Here's how the part is built. I have some questions about the finished solid (model axes, mm). Face numbers are marked on the shaded views. A direction names the side the tool comes from. Give positions to 0.01 mm unless a question says otherwise; leave off trailing zeros. Loops run counter-clockwise (first coordinate to the right, second up) from the corner with the lowest first, then second, coordinate; pieces in that order, holes last. Notation, with made-up numbers: (-13.5, 6.5) - (4.5, 6.5) arc R19 ccw to (4.5, 37.5) - close; hole circle Ø2 at (-7, -7). An arc over 180 degrees is marked (long way). Use a Markdown table: item, result.
from build123d import *

# Parameters (mm, degrees)
SKETCH1_R           = 25
SKETCH1_R_2         = 3
BOSS_EXTRUDE1_DEPTH = 12.5
CUT_EXTRUDE2_DEPTH  = 10
CUT_EXTRUDE3_START  = -4.5
SKETCH2_4_R         = 35
SKETCH2_4_R_2       = 25
CUT_EXTRUDE3_DEPTH  = 17


with BuildPart() as part:
    # Sketch1 → Boss-Extrude1 (new, symmetric)
    with BuildSketch(Plane.XY):
        with BuildLine():
            Line((-33, -40), (33, -40))
            ThreePointArc((33, -40), (37.949747468, -37.949747468), (40, -33))
            Line((40, -33), (40, 33))
            ThreePointArc((40, 33), (37.949747468, 37.949747468), (33, 40))
            Line((33, 40), (-33, 40))
            ThreePointArc((-33, 40), (-37.949747468, 37.949747468), (-40, 33))
            Line((-40, 33), (-40, -33))
            ThreePointArc((-40, -33), (-37.949747468, -37.949747468), (-33, -40))
        make_face()
        Circle(SKETCH1_R, mode=Mode.SUBTRACT)
        with Locations((-33, 33)):
            Circle(SKETCH1_R_2, mode=Mode.SUBTRACT)
        with Locations((33, 33)):
            Circle(SKETCH1_R_2, mode=Mode.SUBTRACT)
        with Locations((-33, -33)):
            Circle(SKETCH1_R_2, mode=Mode.SUBTRACT)
        with Locations((33, -33)):
            Circle(SKETCH1_R_2, mode=Mode.SUBTRACT)
    extrude(amount=BOSS_EXTRUDE1_DEPTH, both=True)

    # Sketch2 → Cut-Extrude2 (cut, symmetric)
    with BuildSketch(Plane.XY):
        with BuildLine():
            Line((-40, 33), (-40, 14.361406616))
            ThreePointArc((-40, 14.361406616), (-30.0520382, 30.0520382), (-14.361406616, 40))
            Line((-14.361406616, 40), (-33, 40))
            ThreePointArc((-33, 40), (-37.949747468, 37.949747468), (-40, 33))
        make_face()
        with BuildLine():
            Line((33, 40), (14.361406616, 40))
            ThreePointArc((14.361406616, 40), (30.0520382, 30.0520382), (40, 14.361406616))
            Line((40, 14.361406616), (40, 33))
            ThreePointArc((40, 33), (37.949747468, 37.949747468), (33, 40))
        make_face()
        with BuildLine():
            ThreePointArc((40, -14.361406616), (30.0520382, -30.0520382), (14.361406616, -40))
            Line((14.361406616, -40), (33, -40))
            ThreePointArc((33, -40), (37.949747468, -37.949747468), (40, -33))
            Line((40, -33), (40, -14.361406616))
        make_face()
        with BuildLine():
            ThreePointArc((-14.361406616, -40), (-30.0520382, -30.0520382), (-40, -14.361406616))
            Line((-40, -14.361406616), (-40, -33))
            ThreePointArc((-40, -33), (-37.949747468, -37.949747468), (-33, -40))
            Line((-33, -40), (-14.361406616, -40))
        make_face()
    extrude(amount=CUT_EXTRUDE2_DEPTH, both=True, mode=Mode.SUBTRACT)

    # Sketch2<4> → Cut-Extrude3 (cut)
    with BuildSketch(Plane.XY.offset(CUT_EXTRUDE3_START)):
        Circle(SKETCH2_4_R)
        Circle(SKETCH2_4_R_2, mode=Mode.SUBTRACT)
    extrude(amount=CUT_EXTRUDE3_DEPTH, mode=Mode.SUBTRACT)


solid = part.part
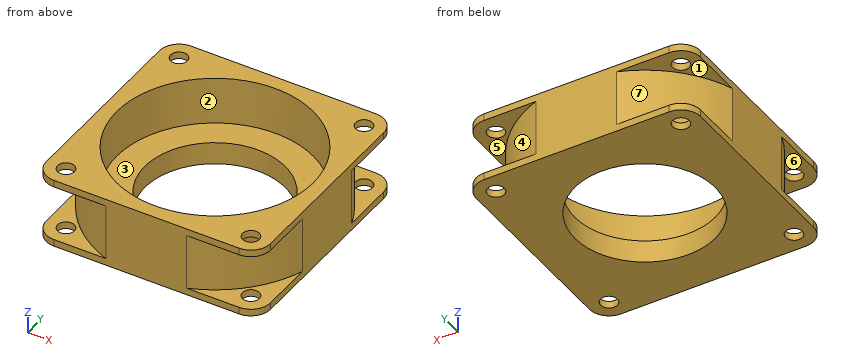
(1) Will these pins go through, and if not, where does the flat tip stop? pin 1 (8 mm diameter, centred on x = 33, y = 33, fed in from -Z); pin 2 (2 mm diameter, centred on y = -24, z = 0.5, fed in from +X); pin 3 (1 mm diameter, centred on y = -27, z = -6.5, fed in from -X); pin 4 (1 mm diameter, centred on y = 15.5, z = -3, fed in from -X).
A:
| item | result |
|---|---|
| pin 1 | z = -12.5 |
| pin 2 | x = 35.74 |
| pin 3 | x = -33.23 |
| pin 4 | x = -39.76 |
(2) On a 3-axis mill with a long thin cutter (end or side, diameter ignored), from which of +Z, -Z, +X, -X, +Y, -Y can I reach the whole of each face in a straight line? I mean the marked faces 5, 6 and 7. Say none if no direction works.
A:
| item | result |
|---|---|
| face 5 | +X, +Y |
| face 6 | -X, -Y |
| face 7 | -X, +Y |
(3) Suppose I cut it at D-D on y = -32. Count the separate pieces of the cut face and the enclosed holes in it, plus the area to 3 significant figures.
A:
| item | result |
|---|---|
| separate pieces | 5 |
| enclosed holes | 0 |
| area | 980 mm2 |
(4) If I drill on line 1 (Y direction, x = 33, z = -11.95); line 2 (Z direction, x = 33.5, y = 26.5), over which ranges is the centre line in solid material (lowest first)?
A:
| item | result |
|---|---|
| line 1 | -40 to -36, -30 to 30, 36 to 40 |
| line 2 | -12.5 to -10, 10 to 12.5 |
(5) Suppose I cut it at C-C on x = 23.5. Write out the boundary of the cut face in (y, z), plus the area to 3 significant figures.
A:
| item | result |
|---|---|
| outline | (-40, -12.5) - (-8.53, -12.5) - (-8.53, -4.5) - (-25.94, -4.5) - (-25.94, 12.5) - (-40, 12.5) - (-40, 10) - (-35.41, 10) - (-35.41, -10) - (-40, -10) - close; (8.53, -12.5) - (40, -12.5) - (40, -10) - (35.41, -10) - (35.41, 10) - (40, 10) - (40, 12.5) - (25.94, 12.5) - (25.94, -4.5) - (8.53, -4.5) - close |
| area | 798 mm2 |
(6) Suppose I cut it at B-B on z = -3. Write out the boundary of the cut face in (x, y), plus the area to 3 significant figures.
A:
| item | result |
|---|---|
| outline | (-40, -14.36) arc R42.5 ccw to (-14.36, -40) - (14.36, -40) arc R42.5 ccw to (40, -14.36) - (40, 14.36) arc R42.5 ccw to (14.36, 40) - (-14.36, 40) arc R42.5 ccw to (-40, 14.36) - close; hole circle Ø70 at (0, 0) |
| area | 1,630 mm2 |
(7) We'd pull the mould along X, two halves only. Please class the marked faces 1, 2, 3 and 4: pulls with the +X half, pulls with the -X half, needs draft (parallel to the pull), parting line crosses it, or undercut.
A:
| item | result |
|---|---|
| face 1 | needs draft |
| face 2 | undercut |
| face 3 | undercut |
| face 4 | pulls with the +X half |
(8) Suppose I cut it at A-A on y = 0. Write out the boundary of the cut face in (x, z).
A:
| item | result |
|---|---|
| outline | (-40, -12.5) - (-25, -12.5) - (-25, -4.5) - (-35, -4.5) - (-35, 12.5) - (-40, 12.5) - close; (25, -12.5) - (40, -12.5) - (40, 12.5) - (35, 12.5) - (35, -4.5) - (25, -4.5) - close |
